```python
from build123d import *

# Parameters (mm, degrees)
F0_R     = 1.55
F0_R_2   = 14.25
F0_R_3   = 1.2
F0_W     = 12
F0_H     = 2
F1_DEPTH = 1.2
F2_DEPTH = 7
F3_R     = 2
F3_R_2   = 1.99999


# Not quite as in the source:
# - a fillet or chamfer is up to 0.001 mm smaller than in the source, because OpenCascade refuses the exact size


with BuildPart() as f1:
    # F0 (on Top) → F1 (new body)
    with BuildSketch(Plane.XY):
        Polygon((12.5, -15), (15, -15), (15, 15), (-15, 15), (-15, -15), (-12.5, -15), (-6, -15), (6, -15), align=None)
        with Locations((-12, -12)):
            Circle(F0_R, mode=Mode.SUBTRACT)
        with Locations((12, -12)):
            Circle(F0_R, mode=Mode.SUBTRACT)
        with Locations((-12, 12)):
            Circle(F0_R, mode=Mode.SUBTRACT)
        Circle(F0_R_2, mode=Mode.SUBTRACT)
        with Locations((12, 12)):
            Circle(F0_R, mode=Mode.SUBTRACT)
        Polygon((-6, -17), (-6, -15), (-12.5, -15), (-12.5, -20), (-6, -20), align=None)
        with Locations((-9.2, -18)):
            Circle(F0_R_3, mode=Mode.SUBTRACT)
        with Locations((0, -16)):
            Rectangle(F0_W, F0_H)
        Polygon((12.5, -20), (12.5, -15), (6, -15), (6, -17), (6, -20), align=None)
        with Locations((9.2, -18)):
            Circle(F0_R_3, mode=Mode.SUBTRACT)
    extrude(amount=F1_DEPTH)

    # F0 (on Top) → F2 (join)
    with BuildSketch(Plane.XY):
        with Locations((0, -16)):
            Rectangle(F0_W, F0_H)
        Polygon((-6, -17), (-6, -15), (-12.5, -15), (-12.5, -20), (-6, -20), align=None)
        with Locations((-9.2, -18)):
            Circle(F0_R_3, mode=Mode.SUBTRACT)
        Polygon((12.5, -20), (12.5, -15), (6, -15), (6, -17), (6, -20), align=None)
        with Locations((9.2, -18)):
            Circle(F0_R_3, mode=Mode.SUBTRACT)
    extrude(amount=F2_DEPTH)

    # F3 (call 1 of 12: OpenCascade refuses the feature's edges together)
    f3_edges = [f1.edges().sort_by_distance(p)[0] for p in [
        (15, -15, 0.6),
    ]]
    fillet(f3_edges, radius=F3_R)

    # F3#2 (call 2 of 12)
    f3_2_edges = [f1.edges().sort_by_distance(p)[0] for p in [
        (-15, -15, 0.6),
    ]]
    fillet(f3_2_edges, radius=F3_R)

    # F3#3 (call 3 of 12)
    f3_3_edges = [f1.edges().sort_by_distance(p)[0] for p in [
        (-15, 15, 0.6),
    ]]
    fillet(f3_3_edges, radius=F3_R)

    # F3#4 (call 4 of 12)
    f3_4_edges = [f1.edges().sort_by_distance(p)[0] for p in [
        (15, 15, 0.6),
    ]]
    fillet(f3_4_edges, radius=F3_R)

    # F3#5 (call 5 of 12)
    f3_5_edges = [f1.edges().sort_by_distance(p)[0] for p in [
        (-12.5, -20, 3.5),
    ]]
    fillet(f3_5_edges, radius=F3_R)

    # F3#6 (call 6 of 12)
    f3_6_edges = [f1.edges().sort_by_distance(p)[0] for p in [
        (-6, -20, 3.5),
    ]]
    fillet(f3_6_edges, radius=F3_R)

    # F3#7 (call 7 of 12)
    f3_7_edges = [f1.edges().sort_by_distance(p)[0] for p in [
        (6, -20, 3.5),
    ]]
    fillet(f3_7_edges, radius=F3_R)

    # F3#8 (call 8 of 12)
    f3_8_edges = [f1.edges().sort_by_distance(p)[0] for p in [
        (12.5, -20, 3.5),
    ]]
    fillet(f3_8_edges, radius=F3_R)

    # F3#9 (call 9 of 12)
    f3_9_edges = [f1.edges().sort_by_distance(p)[0] for p in [
        (12.5, -15, 4.1),
    ]]
    fillet(f3_9_edges, radius=F3_R)

    # F3#10 (call 10 of 12)
    f3_10_edges = [f1.edges().sort_by_distance(p)[0] for p in [
        (-12.5, -15, 4.1),
    ]]
    fillet(f3_10_edges, radius=F3_R)

    # F3#11 (call 11 of 12) (radius 2 in the source; OpenCascade refuses exactly that, so slightly less here)
    f3_11_edges = [f1.edges().sort_by_distance(p)[0] for p in [
        (0, -17, 7),
    ]]
    fillet(f3_11_edges, radius=F3_R_2)

    # F3#12 (call 12 of 12)
    f3_12_edges = [f1.edges().sort_by_distance(p)[0] for p in [
        (0, -17, 0),
    ]]
    fillet(f3_12_edges, radius=F3_R)


solid = f1.part
```
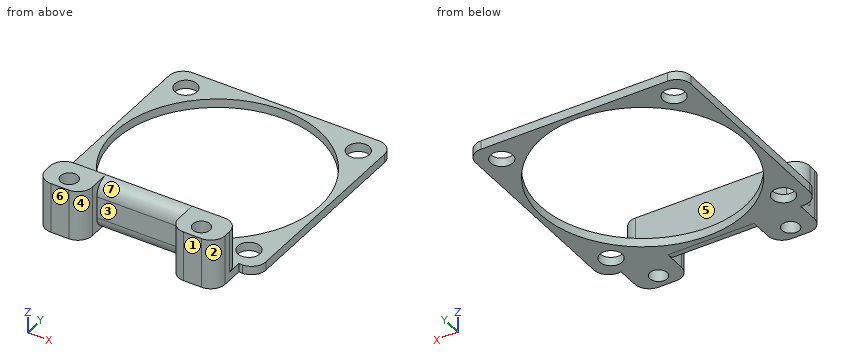
Could you check a few things on this model? Use its own coordinates, in mm. Face numbers are marked on the shaded views. A direction names the side the tool comes from. Round coordinates to 2 decimals unless told otherwise and drop trailing zeros. Loops run counter-clockwise (first coordinate to the right, second up) from the corner with the lowest first, then second, coordinate; pieces in that order, holes last. Notation, with made-up numbers: (9.25, 30.25) -> (54.25, 30.25) arc R16 ccw to (54.25, 53.25) -> close; hole circle Ø9 at (46.5, 3). An arc over 180 degrees is marked (long way). One line per question, with ' | ' between items.
(1) If we section it at B-B on z = 3.5: List the corners of the cut face in (x, y) for me, and give its area (3 significant figures).
Model answer:
outline: (-12.5, -18) arc R2 ccw to (-10.5, -20) -> (-8, -20) arc R2 ccw to (-6, -18) -> (-6, -17) -> (6, -17) -> (6, -18) arc R2 ccw to (8, -20) -> (10.5, -20) arc R2 ccw to (12.5, -18) -> (12.5, -17) arc R2 ccw to (10.5, -15) -> (-10.5, -15) arc R2 ccw to (-12.5, -17) -> close; hole circle Ø2.4 at (-9.2, -18); hole circle Ø2.4 at (9.2, -18) | area: 74.8 mm^2
(2) If we section it at A-A on y = 0: List the corners of the cut face in (x, z) for me.
Model answer:
outline: (-15, 0) -> (-14.25, 0) -> (-14.25, 1.2) -> (-15, 1.2) -> close; (14.25, 0) -> (15, 0) -> (15, 1.2) -> (14.25, 1.2) -> close
(3) Thinking about a two-plate mould opening in X: for the marked faces 1, 2 and 3, which applies, released by +X, released by -X, zero draft, split by the parting line, or undercut?
Model answer:
face 1: zero draft | face 2: released by +X | face 3: undercut
(4) If I drill on probe 1 along Y at (x, z) = (-9.2, 2.5); probe 2 along Y at (x, z) = (12, 0.7); probe 3 along Y at (x, z) = (-10, 0.5), over which ranges is the centre line in solid material (lowest first)?
Model answer:
probe 1: y = -20 to -19.2, -16.8 to -15 | probe 2: y = -19.32 to -13.55, -10.45 to -7.69, 7.69 to 10.45, 13.55 to 15 | probe 3: y = -20 to -18.89, -17.11 to -10.15, 10.15 to 15
(5) For pin 1 Ø3 at (x, y) = (-7, -9.5) entering from -Z; pin 2 Ø2.5 at (y, z) = (-16.5, 2) entering from +X; pin 3 Ø2.5 at (y, z) = (-16.5, 2.5) entering from -X; pin 4 Ø0.6 at (x, z) = (12.5, 0.5) entering from -Y, each with a flat end and sliding along its axis, tell me the tip position at first contact or that it passes through.
Model answer:
pin 1: passes through | pin 2: stops at x = 12.5 | pin 3: stops at x = -12.5 | pin 4: stops at y = -19.05
(6) If we section it at C-C on x = 9.2: List the corners of the cut face in (y, z) for me, and give its area (3 significant figures).
Model answer:
outline: (-20, 0) -> (-19.2, 0) -> (-19.2, 7) -> (-20, 7) -> close; (-16.8, 0) -> (-10.88, 0) -> (-10.88, 1.2) -> (-15, 1.2) -> (-15, 7) -> (-16.8, 7) -> close; (10.88, 0) -> (15, 0) -> (15, 1.2) -> (10.88, 1.2) -> close | area: 28.1 mm^2
(7) For the marked faces 4, 5, 6 and 7, which set-ups out of +Z, -Z, +X, -X, +Y, -Y let a thin tool reach every point of the face, with its end or its side?
Model answer:
face 4: +Z, -Z, -Y | face 5: +Z, +X, -X, +Y | face 6: +Z, -Z, +X, -X, -Y | face 7: +Z, -Y
